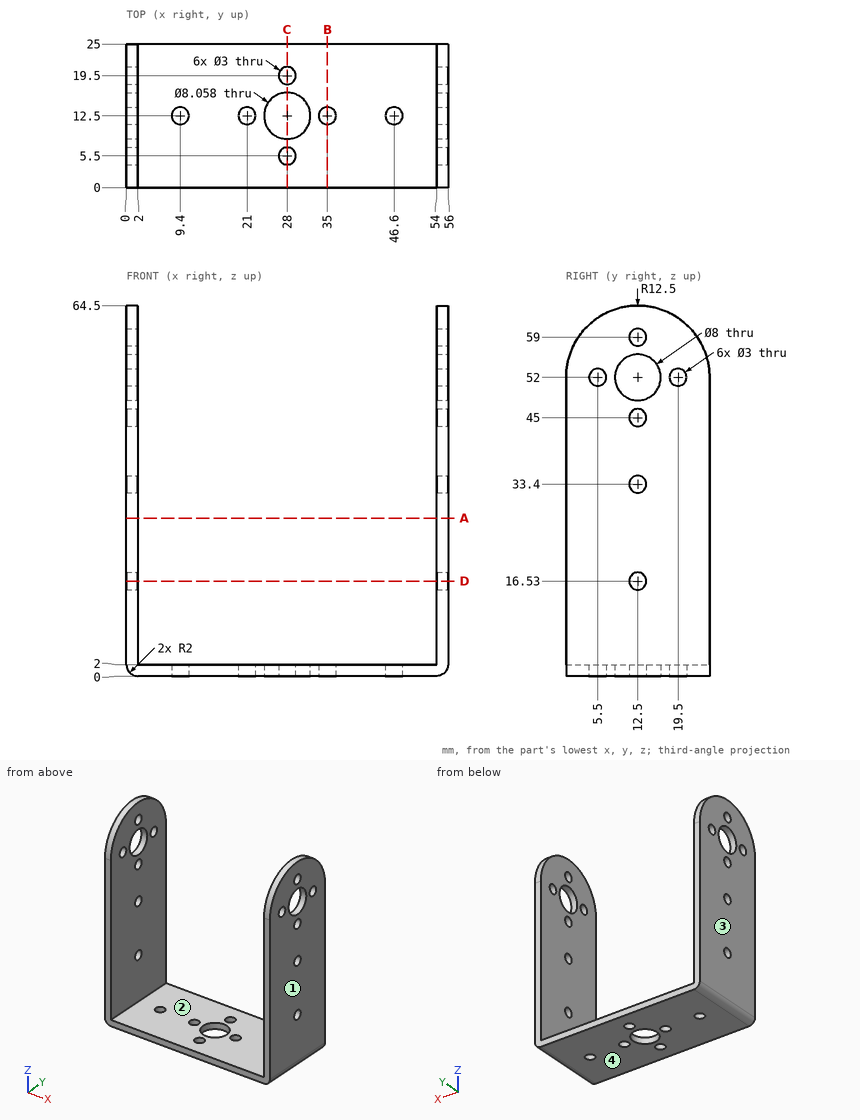
Answer from the drawing. Dimensions are ordinates in mm from the lowest x, y and z of the part. Coordinates: 2 decimals unless noted, no trailing zeros. Write each loop counter-clockwise with the first axis right and the second up, starting at its lowest first coordinate (ties: lowest second). Pieces come first, ordered by that corner, then holes. Notation, with made-up numbers: (4, 34.5) - (41, 34.5) arc R5 cw to (41, 42.5) - close; hole circle Ø8 at (64.25, 82.25). An arc over 180 degrees is marked (long way). One line per question, with ' | ' between items.
Q1. Find section C-C, the plane x = 28. Write down the section's boundary in (y, z), plus the area to 3 significant figures.
Result set:
outline: (0, 0) - (4, 0) - (4, 2) - (0, 2) - close; (7, 0) - (8.47, 0) - (8.47, 2) - (7, 2) - close; (16.53, 0) - (18, 0) - (18, 2) - (16.53, 2) - close; (21, 0) - (25, 0) - (25, 2) - (21, 2) - close | area: 21.9 mm^2
Q2. Consider L1, parallel to X at y = 7, z = 4; L2, parallel to Y at x = 35, z = 0.7; L3, parallel to Z at x = 34, y = 7.5. Determine where each line is inside the solid, lowest interval first. Write a range as [from, to].
Result set:
L1: [0, 2], [54, 56] | L2: [0, 11], [14, 25] | L3: [0, 2]
Q3. Find section B-B, the plane x = 35. Write down the section's boundary in (y, z).
Result set:
outline: (0, 0) - (11, 0) - (11, 2) - (0, 2) - close; (14, 0) - (25, 0) - (25, 2) - (14, 2) - close
Q4. Find section A-A, the plane z = 27.5. Write down the section's boundary in (x, y), plus the area to 3 significant figures.
Result set:
outline: (0, 0) - (2, 0) - (2, 25) - (0, 25) - close; (54, 0) - (56, 0) - (56, 25) - (54, 25) - close | area: 100 mm^2
Q5. Find section D-D, the plane z = 16.53. Write down the section's boundary in (x, y), plus the area to 3 significant figures.
Result set:
outline: (0, 0) - (2, 0) - (2, 11) - (0, 11) - close; (0, 14) - (2, 14) - (2, 25) - (0, 25) - close; (54, 0) - (56, 0) - (56, 11) - (54, 11) - close; (54, 14) - (56, 14) - (56, 25) - (54, 25) - close | area: 88.0 mm^2
Q6. Each of these flat-tipped pins is pushed along its axis until it touches: P1, Ø5, axis at x = 28, y = 12.5, coming from the -Z side; P2, Ø3.5, axis at x = 28, y = 5.5, coming from the +Z side. Where does it stop, or does it pass through?
Result set:
P1: through | P2: z = 2
Q7. Determine the mould class of the marked faces 1, 2, 3 and 4 for opening direction X: +X half, -X half, draft (parallel to the pull), parting line (faces both ways), or undercut.
Result set:
face 1: +X half | face 2: undercut | face 3: -X half | face 4: draft
